Autodesk Inventor part; units mm, degrees
ref_plane "YZ Plane" through (0, 0, 0) normal (1, 0, 0) x (0, 1, 0)
ref_plane "XZ Plane" through (0, 0, 0) normal (0, 1, 0) x (-1, 0, 0)
ref_plane "XY Plane" through (0, 0, 0) normal (0, 0, 1) x (1, 0, 0)
sketch "スケッチ1" plane through (0, 0, 0) normal (1, 0, 0) x (0, 1, 0)
  line L0 (-30, 15) -> (30, 15)
  line L1 (30, 15) -> (30, -15)
  line L2 (30, -15) -> (-30, -15)
  line L3 (-30, -15) -> (-30, 15)
  line L4 (-30, 15) -> (30, -15) construction
  line L5 (30, 15) -> (-30, -15) construction
  line L6 (27.7, -12.7) -> (27.7, 12.7)
  line L7 (27.7, 12.7) -> (-27.7, 12.7)
  line L8 (-27.7, 12.7) -> (-27.7, -12.7)
  line L9 (-27.7, -12.7) -> (27.7, -12.7)
  point P0 (0, 0)
  dimension "d0" = 60
  dimension "d1" = 30
  dimension "d2" = 2.3
extrude "押し出し1" add sketch "スケッチ1" along normal mid plane 34
sketch "スケッチ2" plane through (-17, 30, 15) normal (0, 1, 0) x (1, 0, 0)
  line L0 (0, 0) -> (0, 30)
  circle A0 centre (17, 15) radius 7
  line L1 (34, 0) -> (0, 0)
  point P0 (17, 15)
  dimension "d6" = 14
  dimension "d7" = 17
  dimension "d10" = 15
extrude "押し出し2" cut sketch "スケッチ2" against normal blind 5
sketch "スケッチ3" plane through (-17, -30, 15) normal (0, 0, 1) x (1, 0, 0)
  line L0 (0, 46.9678) -> (20, 46.9678)
  line L1 (20, 46.9678) -> (20, 56.9678)
  line L2 (0, 56.9678) -> (20, 56.9678)
  point P0 (17, 30)
sketch "スケッチ4" plane through (-17, -30, 15) normal (0, 0, 1) x (1, 0, 0)
  circle A0 centre (11, 15) radius 4
  circle A1 centre (11, 35) radius 4
  point P0 (17, 30)
hole "穴1" at (-6, -15, 15) at (-6, 5, 15) direction (0, 0, -1) diameter 8 depth 4 tip angle 118
properties part number "車軸受け2"
Geometry check sheet. Reference: the model listing, model coordinates, mm. A direction names the side the tool comes from. Coordinates: 2 decimals unless noted, no trailing zeros. Loops run counter-clockwise (first coordinate to the right, second up) from the corner with the lowest first, then second, coordinate; pieces in that order, holes last. Notation, with made-up numbers: (88.5, -27) - (147.5, -27) arc R31 cw to (147.5, 8) - close; hole circle Ø7 at (10, 50). An arc over 180 degrees is marked (long way). One line per item, written item: value. Start each with the question number.
(1) Cross-section at C-C on y = 15. Enter the section's corners in (x, z).
(2) Cross-section at D-D on z = 0. Enter the section's corners in (x, y).
(3) Tool access check on faces 1 (the cylindrical face through (6.466, 28.866, 2.681)), 2 (the cylindrical face through (-2.095, 5.867, 13.834)), 3 (the flat face through (0, 0, -12.7)). Record the directions out of +Z, -Z, +X, -X, +Y, -Y that give a thin tool (end or side, any length) a straight path to the whole face; none if there is none.
(4) Depth check by flat-ended pin: P1, Ø5, axis at x = -6, y = 5, coming from the +Z side; P2, Ø11, axis at x = 0, z = 0, coming from the +Y side. Enter the tip coordinate at first touch or a pass-through.
(5) Cross-section at A-A on y = 5. Enter the section's corners in (x, z).
(6) Cross-section at B-B on z = 9.5. Enter the section's corners in (x, y), plus the area to 3 significant figures.
(7) Mould release check, pull along X, two halves, no side actions. Record for faces 4 (the cylindrical face through (-3.6, -11.8, 13.8)), 5 (the flat face through (0, 0, -15)), 6 (the flat face through (17, -2, -13)): released by +X, released by -X, zero draft, split by the parting line, or undercut.
(8) Material ranges on line 1 (Y direction, x = -6, z = 13.2); line 2 (Z direction, x = 0, y = 22); line 3 (Y direction, x = 5.5, z = -4.5), recorded low to high. Write a range as [from, to].
Results below:
1. outline: (-17, -15) - (17, -15) - (17, -12.7) - (-17, -12.7) - close; (-17, 12.7) - (17, 12.7) - (17, 15) - (-17, 15) - close
2. outline: (-17, -30) - (17, -30) - (17, -27.7) - (-17, -27.7) - close; (-17, 27.7) - (-7, 27.7) - (-7, 30) - (-17, 30) - close; (7, 27.7) - (17, 27.7) - (17, 30) - (7, 30) - close
3. face 1: +Y
3. face 2: +Z
3. face 3: +X, -X
4. P1: stops at z = -12.7
4. P2: stops at y = -27.7
5. outline: (-17, -15) - (17, -15) - (17, -12.7) - (-17, -12.7) - close; (-17, 12.7) - (-10, 12.7) - (-10, 15) - (-17, 15) - close; (-2, 12.7) - (17, 12.7) - (17, 15) - (-2, 15) - close
6. outline: (-17, -30) - (17, -30) - (17, -27.7) - (-17, -27.7) - close; (-17, 27.7) - (17, 27.7) - (17, 30) - (-17, 30) - close
6. area: 156 mm2
7. face 4: undercut
7. face 5: zero draft
7. face 6: released by +X
8. line 1: y = [-30, -19], [-11, 1], [9, 30]
8. line 2: z = [-15, -12.7], [12.7, 15]
8. line 3: y = [-30, -27.7], [27.7, 30]
